Could you check a few things on this model? Use its own coordinates, in mm. Give positions to 0.01 mm unless a question says otherwise; leave off trailing zeros. Loops run counter-clockwise (first coordinate to the right, second up) from the corner with the lowest first, then second, coordinate; pieces in that order, holes last. Notation, with made-up numbers: M -33,-37.5 L 22,-37.5 A33 cw 22,-8.5 Z; hole C 58,54 d4. An arc over 180 degrees is marked long. Answer in a Markdown table with one row per item. Add a question column.
1. If we section it at C-C on y = 3.9: Count the separate pieces of the cut face and the enclosed holes in it, then the cut area to 3 significant figures.
2. I need wall thicknesses on line 1 along X through (y, z) = (4.15, 48); line 2 along Z through (x, y) = (25.5, 1.7); line 3 along Z through (x, y) = (-23, 4.5). Which ranges of each line are inside material? Lowest first, please. Write a range as from..to.
3. I'm going to push flat-ended pins straight in: pin 1 Ø1.5 at (x, y) = (-27, 2.5) entering from -Z; pin 2 Ø3 at (y, z) = (4, -65) entering from +X; pin 3 Ø3 at (y, z) = (3.5, -64) entering from -X; pin 4 Ø4 at (x, z) = (23, -48) entering from -Y. Where does each tip first touch, or does it pass through?
4. If we section it at D-D on z = 21.5: List the corners of the cut face in (x, y) for me.
5. If we section it at B-B on x = 26.5: List the corners of the cut face in (y, z) for me, then the cut area to 3 significant figures.
6. If we section it at A-A on z = 48: List the corners of the cut face in (x, y) for me, then the cut area to 3 significant figures.
```python
from build123d import *

# Parameters (mm, degrees)
ESQUISSE1_W             = 60
ESQUISSE1_H             = 122.76
BOSS_EXTRU_1_DEPTH      = 6
ESQUISSE2_W             = 20
ESQUISSE2_H             = 6
BOSS_EXTRU_2_DEPTH      = 6
ESQUISSE3_R             = 1.5
ENL_V_MAT_EXTRU_1_DEPTH = 6
ESQUISSE4_W             = 5
ESQUISSE4_H             = 35
ENL_V_MAT_EXTRU_2_DEPTH = 6


with BuildPart() as part:
    # Esquisse1 → Boss.-Extru.1 (new body)
    with BuildSketch(Plane(origin=(0, 0, 0), x_dir=(1, 0, 0), z_dir=(0, 1, 0))):
        Rectangle(ESQUISSE1_W, ESQUISSE1_H)
    extrude(amount=BOSS_EXTRU_1_DEPTH)

    # Esquisse2 → Boss.-Extru.2 (add)
    with BuildSketch(Plane(origin=(0, 6, 0), x_dir=(1, 0, 0), z_dir=(0, 1, 0))):
        with Locations((-15, 64.38)):
            Rectangle(ESQUISSE2_W, ESQUISSE2_H)
        with Locations((15, 64.38)):
            Rectangle(ESQUISSE2_W, ESQUISSE2_H)
        with Locations((15, -64.38)):
            Rectangle(ESQUISSE2_W, ESQUISSE2_H)
        with Locations((-15, -64.38)):
            Rectangle(ESQUISSE2_W, ESQUISSE2_H)
    extrude(amount=-BOSS_EXTRU_2_DEPTH)

    # Esquisse3 → Enlèv. mat.-Extru.1 (cut)
    with BuildSketch(Plane(origin=(0, 6, 0), x_dir=(1, 0, 0), z_dir=(0, 1, 0))):
        with Locations((23, 48)):
            Circle(ESQUISSE3_R)
        with Locations((-23, 48)):
            Circle(ESQUISSE3_R)
        with Locations((-23, -48)):
            Circle(ESQUISSE3_R)
        with Locations((23, -48)):
            Circle(ESQUISSE3_R)
    extrude(amount=-ENL_V_MAT_EXTRU_1_DEPTH, mode=Mode.SUBTRACT)

    # Esquisse4 → Enlèv. mat.-Extru.2 (cut)
    with BuildSketch(Plane(origin=(0, 6, 0), x_dir=(1, 0, 0), z_dir=(0, 1, 0))):
        with Locations((-27.5, -20.88)):
            Rectangle(ESQUISSE4_W, ESQUISSE4_H)
        with Locations((27.5, -20.88)):
            Rectangle(ESQUISSE4_W, ESQUISSE4_H)
        with Locations((-27.5, 20.88)):
            Rectangle(ESQUISSE4_W, ESQUISSE4_H)
        with Locations((27.5, 20.88)):
            Rectangle(ESQUISSE4_W, ESQUISSE4_H)
    extrude(amount=-ENL_V_MAT_EXTRU_2_DEPTH, mode=Mode.SUBTRACT)


solid = part.part
```
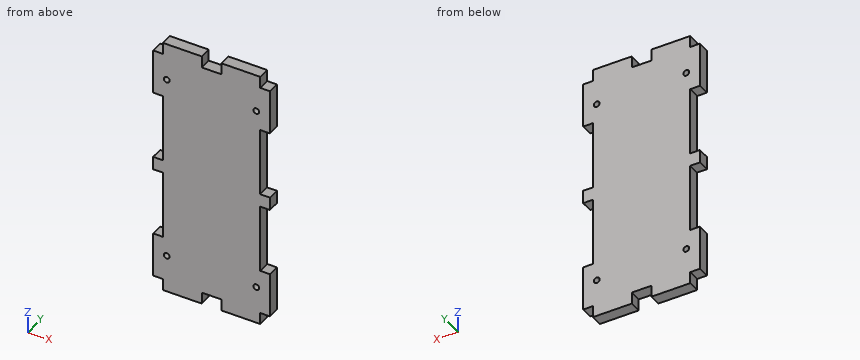
Results:
| question | item | result |
|---|---|---|
| 1 | separate pieces | 1 |
| 1 | enclosed holes | 4 |
| 1 | area | 7,120 mm2 |
| 2 | line 1 | -30..-24.5, -21.5..21.5, 24.5..30 |
| 2 | line 2 | -61.38..-38.38, -3.38..3.38, 38.38..61.38 |
| 2 | line 3 | -67.38..-49.5, -46.5..46.5, 49.5..67.38 |
| 3 | pin 1 | z = -61.38 |
| 3 | pin 2 | x = 25 |
| 3 | pin 3 | x = -25 |
| 3 | pin 4 | y = 0 |
| 4 | outline | M -25,0 L 25,0 L 25,6 L -25,6 Z |
| 5 | outline | M 0,-61.38 L 6,-61.38 L 6,-38.38 L 0,-38.38 Z; M 0,-3.38 L 6,-3.38 L 6,3.38 L 0,3.38 Z; M 0,38.38 L 6,38.38 L 6,61.38 L 0,61.38 Z |
| 5 | area | 317 mm2 |
| 6 | outline | M -30,0 L -24.5,0 L -24.5,6 L -30,6 Z; M -21.5,0 L 21.5,0 L 21.5,6 L -21.5,6 Z; M 24.5,0 L 30,0 L 30,6 L 24.5,6 Z |
| 6 | area | 324 mm2 |
